from build123d import *

# Parameters (mm, degrees)
BOSS_EXTRUDE1_DEPTH = 20
FILLET1_R           = 8
SKETCH2_W           = 25.416334399
SKETCH2_H           = 26.69942318
CUT_EXTRUDE1_DEPTH  = 14
SKETCH3_R           = 2.920242488
CUT_EXTRUDE2_DEPTH  = 7
SKETCH4_R           = 8.768125441
BOSS_EXTRUDE2_DEPTH = 21.004475


with BuildPart() as part:
    # Sketch1 → Boss-Extrude1 (new body)
    with BuildSketch(Plane(origin=(0, 0, 0), x_dir=(1, 0, 0), z_dir=(0, 1, 0))):
        Polygon((-61.131192742, -32.931354604), (72.486832261, -32.931354604), (72.486832261, -24.982406941), (51.482357687, -24.982406941), (51.482357687, 25.600715877), (72.486832261, 25.600715877), (72.486832261, 43.529951488), (-61.131192742, 43.529951488), (-61.131192742, 35.202482508), (-53.52918853, 35.202482508), (-53.52918853, -24.982406941), (-61.131192742, -24.982406941), align=None)
    extrude(amount=BOSS_EXTRUDE1_DEPTH)

    # Fillet1
    fillet1_edges = [part.edges().sort_by_distance(p)[0] for p in [
        (72.486832261, 10, -43.529951488),
        (72.486832261, 10, -25.600715877),
    ]]
    fillet(fillet1_edges, radius=FILLET1_R)

    # Sketch2 → Cut-Extrude1 (cut)
    with BuildSketch(Plane(origin=(0, 20, 0), x_dir=(1, 0, 0), z_dir=(0, 1, 0))):
        with Locations((64.190524887, 34.382431467)):
            Rectangle(SKETCH2_W, SKETCH2_H)
    extrude(amount=-CUT_EXTRUDE1_DEPTH, mode=Mode.SUBTRACT)

    # Sketch3 → Cut-Extrude2 (cut, through all)
    with BuildSketch(Plane(origin=(0, 6, 0), x_dir=(1, 0, 0), z_dir=(0, 1, 0))):
        with Locations(Location((62.010238624, 35.19513013, 0), (0, 0, 270))):  # turned: the seam where the file's is
            Circle(SKETCH3_R)
    extrude(amount=-CUT_EXTRUDE2_DEPTH, mode=Mode.SUBTRACT)

    # Sketch4 → Boss-Extrude2 (add)
    with BuildSketch(Plane(origin=(51.482357687, 0, 0), x_dir=(0, 0, -1), z_dir=(1, 0, 0))):
        with Locations(Location((9.656027264, 9.243975153, 0), (0, 0, 180))):  # turned: the seam where the file's is
            Circle(SKETCH4_R)
    extrude(amount=BOSS_EXTRUDE2_DEPTH)


solid = part.part
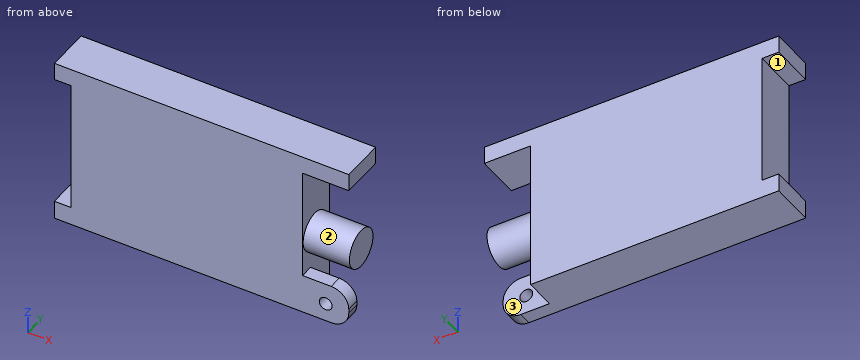
Work out the finished part from the listing and answer in its coordinate system (mm). Face numbers are marked on the shaded views. A direction names the side the tool comes from. Round coordinates to 2 decimals unless told otherwise and drop trailing zeros. Write each loop counter-clockwise with the first axis right and the second up, starting at its lowest first coordinate (ties: lowest second). Pieces come first, ordered by that corner, then holes. Notation, with made-up numbers: (19, -17.5) - (30, -17.5) arc R18 cw to (30, 16.5) - close; hole circle Ø10 at (-25.5, 73). An arc over 180 degrees is marked (long way). Answer in a Markdown table with one row per item. Add a question column.
1. Find the intervals of material crossed by line 1 along X through (y, z) = (1, -2); line 2 along Y through (x, z) = (62, -38.5); line 3 along X through (y, z) = (2, -14), in increasing order. Write a range as from..to.
2. For the marked faces 1, 2 and 3, determine the directions among +Z, -Z, +X, -X, +Y, -Y from which every point of the face is accessible in a straight line to the end or side of a thin tool.
3. Given pin 1 (3 mm diameter, centred on y = 14, z = 19.5, fed in from +X); pin 2 (1 mm diameter, centred on y = 15, z = 12.5, fed in from -X); pin 3 (9 mm diameter, centred on x = 62, z = -38.5, fed in from +Y), each flat-ended and moving along its own axis, determine where each tip first touches the part or whether it passes through.
4. A cutting plane is placed at B-B, the plane z = 20.5. Determine the outline of the cut face in (x, y).
5. A cutting plane is placed at D-D, the plane z = -4.5. Determine the outline of the cut face in (x, y).
6. A cutting plane is placed at C-C, the plane y = 13.75. Determine the outline of the cut face in (x, z), and give its area (3 significant figures).
7. A cutting plane is placed at A-A, the plane y = 2.5. Determine the outline of the cut face in (x, z), and give its area (3 significant figures).
Worked out:
| question | item | result |
|---|---|---|
| 1 | line 1 | -53.53..51.48 |
| 1 | line 2 | 0..6 |
| 1 | line 3 | -53.53..72.49 |
| 2 | face 1 | -X, +Y, -Y |
| 2 | face 2 | +X |
| 2 | face 3 | -Z, +X, +Y |
| 3 | pin 1 | x = 51.48 |
| 3 | pin 2 | x = -53.53 |
| 3 | pin 3 | y = 6 |
| 4 | outline | (-53.53, 0) - (51.48, 0) - (51.48, 20) - (-53.53, 20) - close |
| 5 | outline | (-53.53, 0) - (51.48, 0) - (51.48, 2.15) - (72.49, 2.15) - (72.49, 16.34) - (51.48, 16.34) - (51.48, 20) - (-53.53, 20) - close |
| 6 | outline | (-61.13, -43.53) - (51.48, -43.53) - (51.48, -17.18) - (72.49, -17.18) - (72.49, -2.13) - (51.48, -2.13) - (51.48, 24.98) - (72.49, 24.98) - (72.49, 32.93) - (-61.13, 32.93) - (-61.13, 24.98) - (-53.53, 24.98) - (-53.53, -35.2) - (-61.13, -35.2) - close |
| 6 | area | 8,640 mm^2 |
| 7 | outline | (-61.13, -43.53) - (64.49, -43.53) arc R8 ccw to (72.49, -35.53) - (72.49, -33.6) arc R8 ccw to (64.49, -25.6) - (51.48, -25.6) - (51.48, -15.26) - (72.49, -15.26) - (72.49, -4.05) - (51.48, -4.05) - (51.48, 24.98) - (72.49, 24.98) - (72.49, 32.93) - (-61.13, 32.93) - (-61.13, 24.98) - (-53.53, 24.98) - (-53.53, -35.2) - (-61.13, -35.2) - close; hole circle Ø5.84 at (62.01, -35.2) |
| 7 | area | 8,880 mm^2 |
